Autodesk Inventor part; units mm, degrees
ref_plane "YZ Plane" through (0, 0, 0) normal (1, 0, 0) x (0, 1, 0)
ref_plane "XZ Plane" through (0, 0, 0) normal (0, 1, 0) x (-1, 0, 0)
ref_plane "XY Plane" through (0, 0, 0) normal (0, 0, 1) x (1, 0, 0)
sketch "Sketch1" plane through (0, 0, 0) normal (0, 0, 1) x (1, 0, 0)
  line L0 (0, 0) -> (85, 0)
  line L1 (85, 0) -> (85, -56)
  line L2 (85, -56) -> (0, -56)
  line L3 (0, -56) -> (0, 0)
  dimension "d0" = 85
  dimension "d1" = 56
extrude "Extrusion1" add sketch "Sketch1" along normal blind 1
fillet "Congé1" radius 3 4 edges at (0, 0, 0.5) (85, 0, 0.5) (85, -56, 0.5) (0, -56, 0.5)
sketch "Esquisse2" plane through (0, 0, 1) normal (0, 0, 1) x (1, 0, 0)
  point P0 (0, 0)
sketch "Esquisse3" plane through (0, 0, 1) normal (0, 0, 1) x (1, 0, 0)
  arc A0 (0, -53) -> (3, -56) centre (3, -53) ccw construction
  line L0 (3, -56) -> (82, -56) construction
  arc A1 (82, -56) -> (85, -53) centre (82, -53) ccw construction
  line L1 (85, -53) -> (85, -3) construction
  arc A2 (85, -3) -> (82, 0) centre (82, -3) ccw construction
  line L2 (82, 0) -> (3, 0) construction
  arc A3 (3, 0) -> (0, -3) centre (3, -3) ccw construction
  line L3 (0, -3) -> (0, -53) construction
  line L4 (3.5, -3.5) -> (61.5, -3.5) construction
  line L5 (61.5, -3.5) -> (61.5, -52.5) construction
  line L6 (61.5, -52.5) -> (3.5, -52.5) construction
  line L7 (3.5, -52.5) -> (3.5, -3.5) construction
  point P0 (0, 0)
  dimension "d5" = 3.5
  dimension "d6" = 49
  dimension "d7" = 58
  dimension "d8" = 3.5
hole "Perçage1" at (61.5, -52.5, 1) at (3.5, -52.5, 1) at (3.5, -3.5, 1) at (61.5, -3.5, 1) direction (0, 0, -1) diameter 3 end through all
properties part number "R000"
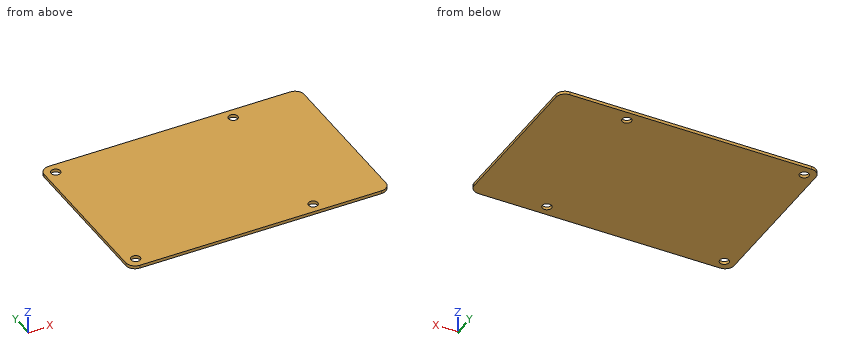
Could you check a few things on this model? Use its own coordinates, in mm. Give positions to 0.01 mm unless a question says otherwise; leave off trailing zeros. Write each loop counter-clockwise with the first axis right and the second up, starting at its lowest first coordinate (ties: lowest second). Pieces come first, ordered by that corner, then holes. Notation, with made-up numbers: (-9.5, 82.25) -> (43.5, 82.25) arc R6 ccw to (43.5, 90.25) -> close; hole circle Ø8 at (6, 54.5). An arc over 180 degrees is marked (long way). Answer as a JSON object with one key per item and string values.
Q1. Suppose I cut it at A-A on x = 61.5. Write out the boundary of the cut face in (y, z).
Taken from the geometry:
{"outline": "(-56, 0) -> (-54, 0) -> (-54, 1) -> (-56, 1) -> close; (-51, 0) -> (-5, 0) -> (-5, 1) -> (-51, 1) -> close; (-2, 0) -> (0, 0) -> (0, 1) -> (-2, 1) -> close"}
Q2. Please list where these lines run through material, in increasing order: L1, parallel to X at y = -3.5, z = 0.7; L2, parallel to Y at x = 61.5, z = 0.75; L3, parallel to Y at x = 62.5, z = 0.85.
Taken from the geometry:
{"L1": "x = 0 to 2, 5 to 60, 63 to 85", "L2": "y = -56 to -54, -51 to -5, -2 to 0", "L3": "y = -56 to -53.62, -51.38 to -4.62, -2.38 to 0"}
Q3. Will these pins go through, and if not, where does the flat tip stop? pin 1 Ø1.8 at (x, y) = (3.5, -52.5) entering from +Z; pin 2 Ø1.5 at (x, y) = (76, -10.5) entering from -Z.
Taken from the geometry:
{"pin 1": "passes through", "pin 2": "stops at z = 0"}
